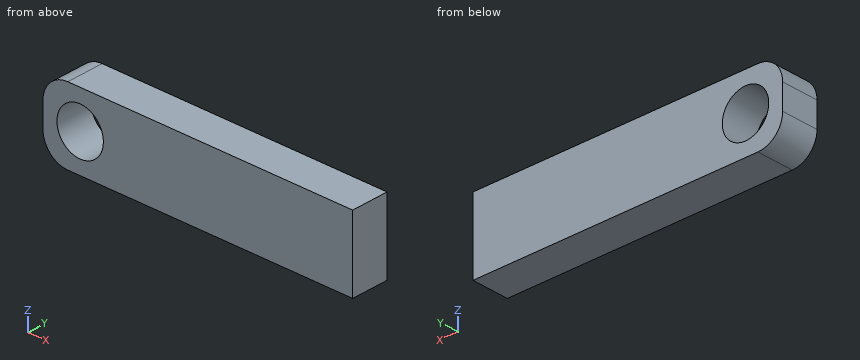
from build123d import *

# Parameters (mm, degrees)
F0_W     = 25
F0_H     = 6
F0_R     = 1.875
F1_DEPTH = 3
F2_R     = 2


with BuildPart() as f1:
    # F0 (on Front) → F1 (new body)
    with BuildSketch(Plane.XZ):
        with Locations((-23.103761, 24.092039)):
            Rectangle(F0_W, F0_H)
        with Locations((-32.603761, 24.092039)):
            Circle(F0_R, mode=Mode.SUBTRACT)
    extrude(amount=F1_DEPTH)

    # F2
    f2_edges = [f1.edges().sort_by_distance(p)[0] for p in [
        (-35.603761, -1.5, 27.092039),
        (-35.603761, -1.5, 21.092039),
    ]]
    fillet(f2_edges, radius=F2_R)


solid = f1.part
Geometry: final body of the model. Coordinates: model frame, mm. Round coordinates to 2 decimals unless told otherwise and drop trailing zeros. Loops run counter-clockwise (first coordinate to the right, second up) from the corner with the lowest first, then second, coordinate; pieces in that order, holes last. Notation, with made-up numbers: (23.5, 26) -> (76.5, 26) arc R18 ccw to (76.5, 51) -> close; hole circle Ø6 at (-7.75, 25). An arc over 180 degrees is marked (long way). One line per question, with ' | ' between items. Start each with the question number.
1. Line query: line 1 along X through (y, z) = (-1.1, 23.1); line 2 along Z through (x, y) = (-32.5, -0.2); line 3 along X through (y, z) = (-2.7, 25.7). Output: solid intervals per line, ascending. Write a range as [from, to].
2. Section C-C on z = 23.3. Output: boundary loops of the cut face in (x, y), and give its area (3 significant figures).
3. Section B-B on y = -0.85. Output: boundary loops of the cut face in (x, z) (3 decimals).
4. Section D-D on z = 21.65. Output: boundary loops of the cut face in (x, y), and give its area (3 significant figures).
5. Section A-A on z = 24.65. Output: boundary loops of the cut face in (x, y), and give its area (3 significant figures).
Returned:
1) line 1: x = [-35.6, -34.19], [-31.01, -10.6] | line 2: z = [21.09, 22.22], [25.96, 27.09] | line 3: x = [-35.51, -33.57], [-31.64, -10.6]
2) outline: (-35.6, -3) -> (-34.3, -3) -> (-34.3, 0) -> (-35.6, 0) -> close; (-30.9, -3) -> (-10.6, -3) -> (-10.6, 0) -> (-30.9, 0) -> close | area: 64.8 mm2
3) outline: (-35.604, 23.092) arc R2 ccw to (-33.604, 21.092) -> (-10.604, 21.092) -> (-10.604, 27.092) -> (-33.604, 27.092) arc R2 ccw to (-35.604, 25.092) -> close; hole circle Ø3.75 at (-32.604, 24.092)
4) outline: (-34.99, -3) -> (-10.6, -3) -> (-10.6, 0) -> (-34.99, 0) -> close | area: 73.2 mm2
5) outline: (-35.6, -3) -> (-34.39, -3) -> (-34.39, 0) -> (-35.6, 0) -> close; (-30.81, -3) -> (-10.6, -3) -> (-10.6, 0) -> (-30.81, 0) -> close | area: 64.3 mm2
